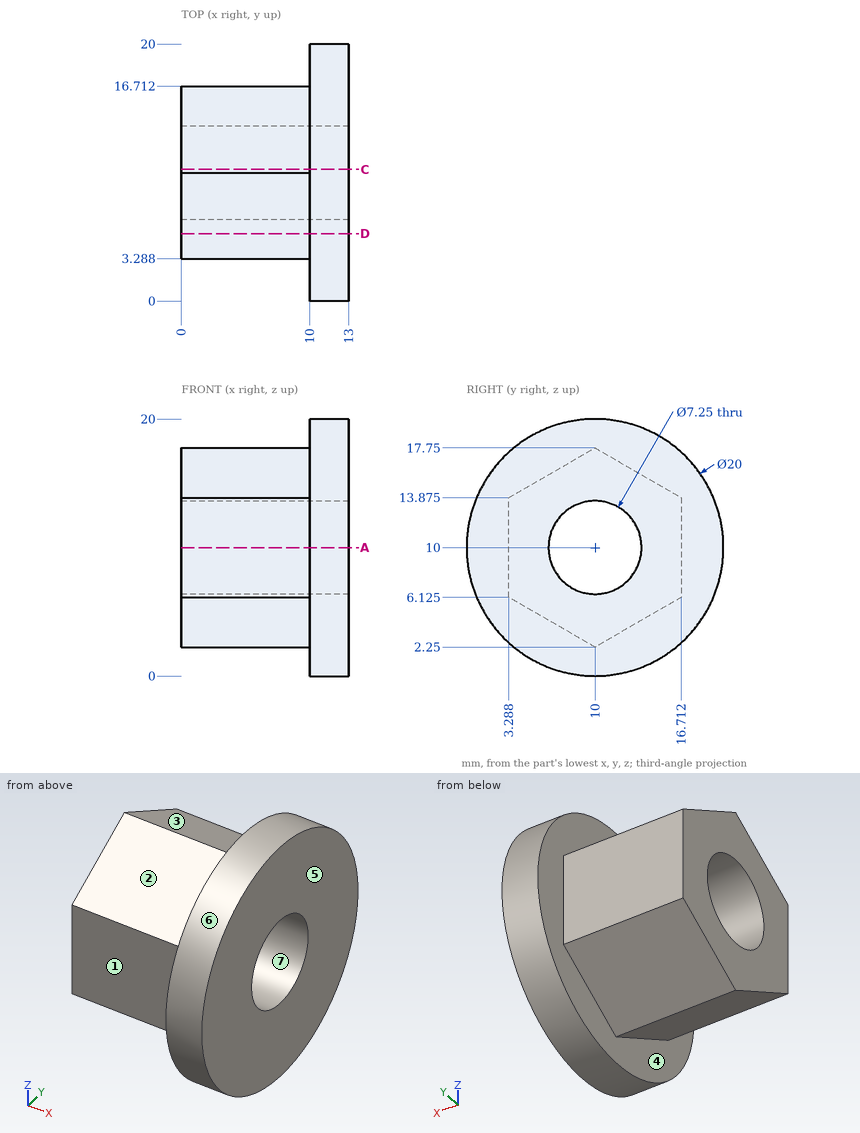
Check sheet for the drawn part. Datum: minimum x, y, z corner. Units: mm. A direction names the side the tool comes from. Coordinates: 2 decimals unless noted, no trailing zeros. Loops run counter-clockwise (first coordinate to the right, second up) from the corner with the lowest first, then second, coordinate; pieces in that order, holes last. Notation, with made-up numbers: (-22.75, 82) -> (33.25, 82) arc R20 cw to (33.25, 112) -> close; hole circle Ø6 at (47.5, 68). An arc over 180 degrees is marked (long way). Answer as CSV lines item,"result".
1) Cross-section at A-A, the plane z = 10. Record the cut outline in (x, y) (1 decimal).
Found:
outline,"(0, 3.3) -> (10, 3.3) -> (10, 0) -> (13, 0) -> (13, 6.4) -> (0, 6.4) -> close; (0, 13.6) -> (13, 13.6) -> (13, 20) -> (10, 20) -> (10, 16.7) -> (0, 16.7) -> close"
2) Cross-section at D-D, the plane y = 5.25. Record the cut outline in (x, z), then the cut area to 3 significant figures.
Found:
outline,"(0, 4.99) -> (10, 4.99) -> (10, 1.2) -> (13, 1.2) -> (13, 18.8) -> (10, 18.8) -> (10, 15.01) -> (0, 15.01) -> close"
area,"153 mm2"
3) Depth check by flat-ended pin: pin 1 (2.5 mm diameter, centred on x = 4.5, z = 10, fed in from +Y); pin 2 (2 mm diameter, centred on x = 6.5, y = 6.5, fed in from -Z); pin 3 (2.5 mm diameter, centred on x = 5, z = 10, fed in from -Y). Enter the tip coordinate at first touch or a pass-through.
Found:
pin 1,"stops at y = 16.71"
pin 2,"stops at z = 3.69"
pin 3,"stops at y = 3.29"
4) Release check for a two-part mould opening along Z. For the marked faces 5, 6 and 7 record: +Z half, -Z half, draft (parallel to the pull), parting line (faces both ways), or undercut.
Found:
face 5,"draft"
face 6,"parting line"
face 7,"undercut"
5) Tool access check on the marked faces 1, 2, 3 and 4. Record the directions out of +Z, -Z, +X, -X, +Y, -Y that give a thin tool (end or side, any length) a straight path to the whole face; none if there is none.
Found:
face 1,"+Z, -Z, -X, -Y"
face 2,"+Z, -X, -Y"
face 3,"+Z, -X, +Y"
face 4,"-X"
6) Thickness scan on L1, parallel to Y at x = 9.75, z = 10 (1 decimal); L2, parallel to X at y = 6.5, z = 3.25; L3, parallel to Z at x = 1.25, y = 11.75 (1 decimal). Record the ranges inside material, lowest first. Write a range as from..to.
Found:
L1,"y = 3.3..6.4, 13.6..16.7"
L2,"x = 10..13"
L3,"z = 3.3..6.8, 13.2..16.7"
7) Cross-section at C-C, the plane y = 10.25. Record the cut outline in (x, z).
Found:
outline,"(0, 2.39) -> (10, 2.39) -> (10, 0) -> (13, 0) -> (13, 6.38) -> (0, 6.38) -> close; (0, 13.62) -> (13, 13.62) -> (13, 20) -> (10, 20) -> (10, 17.61) -> (0, 17.61) -> close"
